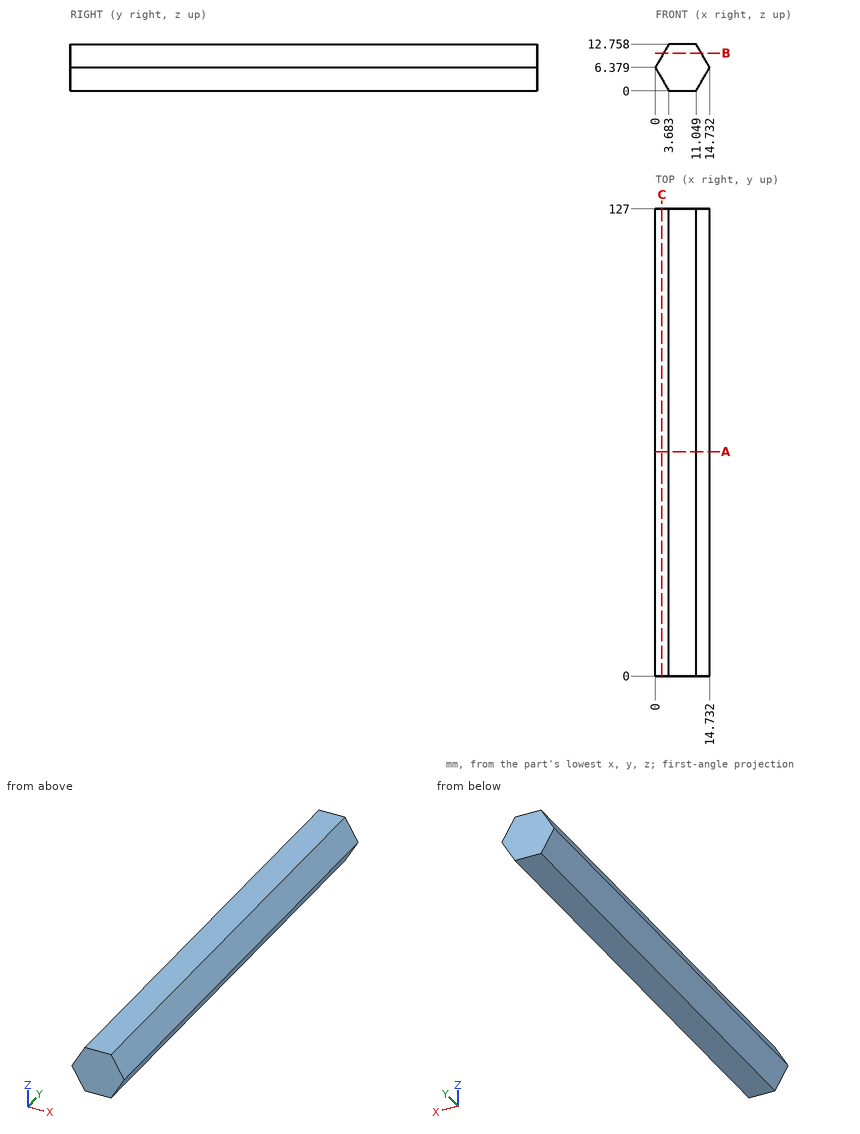
The drawing under review shows one solid part. Ordinate dimensions are in mm from its lowest x, y, z. Round coordinates to 2 decimals unless told otherwise and drop trailing zeros. Write each loop counter-clockwise with the first axis right and the second up, starting at its lowest first coordinate (ties: lowest second). Pieces come first, ordered by that corner, then holes. Notation, with made-up numbers: (-30, -10.5) -> (19, -10.5) arc R21 ccw to (19, 26.5) -> close; hole circle Ø5 at (15.5, 56.25). An arc over 180 degrees is marked (long way). One line per question, with ' | ' between items. Start each with the question number.
(1) Add section C-C, the plane x = 1.75. Write out the cut boundary in (y, z), plus the area to 3 significant figures.
(2) Add section A-A, the plane y = 61. Write out the cut boundary in (x, z), plus the area to 3 significant figures.
(3) For line 1 along Z through (x, y) = (1.5, 73); line 2 along Z through (x, y) = (1, 102); line 3 along X through (y, z) = (55, 8.5) (1 decimal), list the stretches that pass through material, from the lowest coordinate up. Write a range as from..to.
(4) Insertion check: P1, Ø2, axis at y = 99, z = 8, coming from the +X side; P2, Ø3, axis at y = 67, z = 10, coming from the -X side (1 decimal); P3, Ø1, axis at x = 1.5, y = 19.5, coming from the -Z side (1 decimal). Each pin has a flat end and moves straight along its axis. Give the tip position at first contact, or say it passes through.
(5) Add section B-B, the plane z = 10.25. Write out the cut boundary in (x, y) (1 decimal), plus the area to 3 significant figures.
Answer list:
1) outline: (0, 3.35) -> (127, 3.35) -> (127, 9.41) -> (0, 9.41) -> close | area: 770 mm²
2) outline: (0, 6.38) -> (3.68, 0) -> (11.05, 0) -> (14.73, 6.38) -> (11.05, 12.76) -> (3.68, 12.76) -> close | area: 141 mm²
3) line 1: 3.78..8.98 | line 2: 4.65..8.11 | line 3: 1.2..13.5
4) P1: x = 14.37 | P2: x = 1.2 | P3: z = 2.9
5) outline: (2.2, 0) -> (12.5, 0) -> (12.5, 127) -> (2.2, 127) -> close | area: 1,300 mm²
